Geometry check sheet. Reference: drawing and pictorial views, mm from the part's lowest x, y, z. A direction names the side the tool comes from. Give positions to 0.01 mm unless a question says otherwise; leave off trailing zeros. Order: outer loops, then holes, each group sorted by start corner. A loop starts at its lowest first (then second) coordinate and runs counter-clockwise, first axis right, second up.
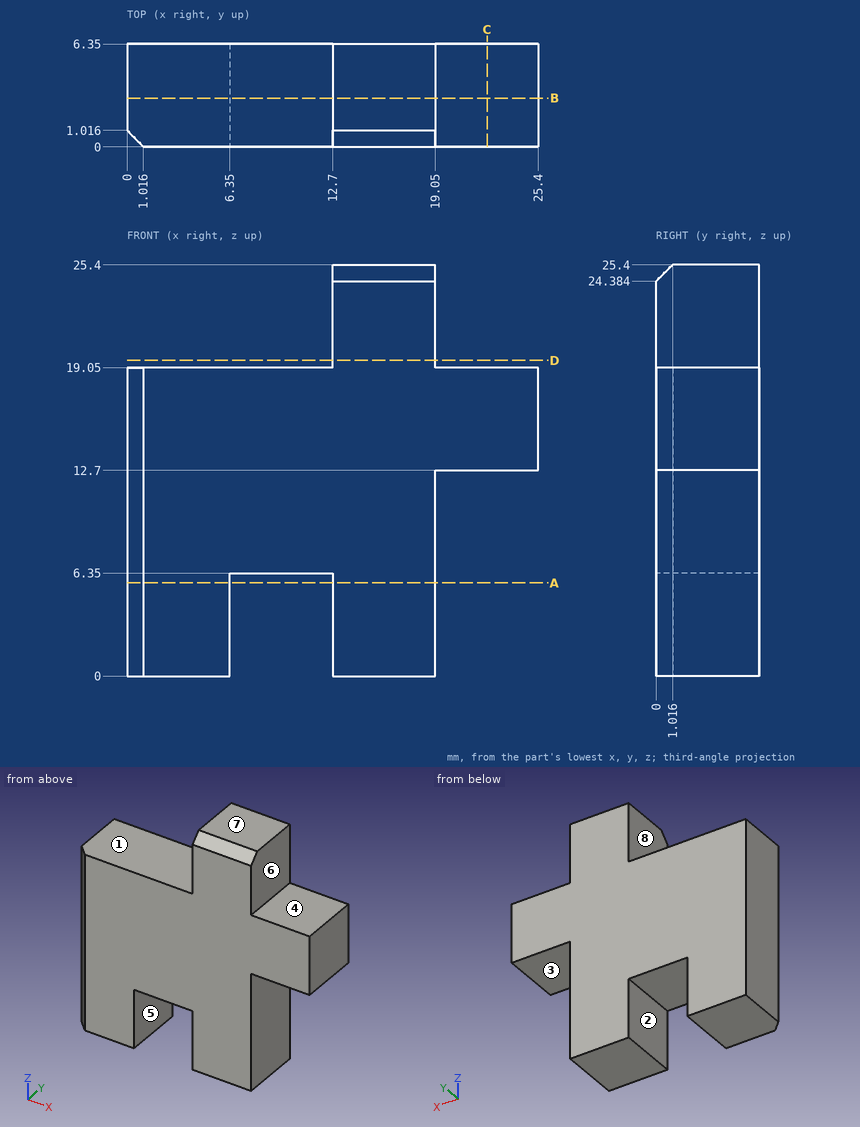
1) Depth check by flat-ended pin: pin 1 Ø1.9 at (y, z) = (2, 8.5) entering from +X; pin 2 Ø1.9 at (x, y) = (21, 4) entering from +Z; pin 3 Ø1.9 at (y, z) = (4.5, 23.5) entering from -X. Enter the tip coordinate at first touch or a pass-through.
Recorded:
pin 1: stops at x = 19.05
pin 2: stops at z = 19.05
pin 3: stops at x = 12.7
2) Draft check along X on the marked faces 5, 6, 7 and 8. Enter one of: +X half, -X half, draft (parallel to the pull), parting line (faces both ways), or undercut.
Recorded:
face 5: undercut
face 6: +X half
face 7: draft
face 8: -X half
3) Section check B-B, the plane y = 3. Record the cut outline in (x, z).
Recorded:
outline: (0, 0) - (6.35, 0) - (6.35, 6.35) - (12.7, 6.35) - (12.7, 0) - (19.05, 0) - (19.05, 12.7) - (25.4, 12.7) - (25.4, 19.05) - (19.05, 19.05) - (19.05, 25.4) - (12.7, 25.4) - (12.7, 19.05) - (0, 19.05) - close
4) Section check A-A, the plane z = 5.75. Record the cut outline in (x, y), then the cut area to 3 significant figures.
Recorded:
outline: (0, 1.02) - (1.02, 0) - (6.35, 0) - (6.35, 6.35) - (0, 6.35) - close; (12.7, 0) - (19.05, 0) - (19.05, 6.35) - (12.7, 6.35) - close
area: 80.1 mm2
5) Section check C-C, the plane x = 22.25. Record the cut outline in (y, z).
Recorded:
outline: (0, 12.7) - (6.35, 12.7) - (6.35, 19.05) - (0, 19.05) - close
6) Section check D-D, the plane z = 19.5. Record the cut outline in (x, y).
Recorded:
outline: (12.7, 0) - (19.05, 0) - (19.05, 6.35) - (12.7, 6.35) - close
7) Material ranges on L1, parallel to X at y = 2, z = 6; L2, parallel to Z at x = 23.25, y = 5.75; L3, parallel to Z at x = 12.5, y = 6.25, recorded low to high.
Recorded:
L1: x = 0 to 6.35, 12.7 to 19.05
L2: z = 12.7 to 19.05
L3: z = 6.35 to 19.05
8) Set-up check for the marked faces 1, 2, 3 and 4: record each of +Z, -Z, +X, -X, +Y, -Y from which the full face is reachable in a straight line by a thin tool's end or side.
Recorded:
face 1: +Z, -X, +Y, -Y
face 2: -Z, +Y, -Y
face 3: -Z, +X, +Y, -Y
face 4: +Z, +X, +Y, -Y
